from build123d import *

# Parameters (mm, degrees)
CYLINDER001_R         = 1.5
CYLINDER001_DEPTH     = 10
SKETCH002_W           = 15
SKETCH002_H           = 26
PAD_DEPTH             = 10
CLONE_SCALE_SCALE     = 2
CLONE_PLACEMENT_ANGLE = 90
BOX_W                 = 6
BOX_H                 = 20
BOX_DEPTH             = 10


with BuildPart() as obj1:
    # Cylinder001 → Cylinder001 (new body)
    with BuildSketch(Plane.XY.offset(114)):
        Circle(CYLINDER001_R)
    extrude(amount=CYLINDER001_DEPTH)


with BuildPart() as nul:
    # Sketch002 → Pad (new body)
    with BuildSketch(Plane.XY.offset(11.4)):
        with BuildLine():
            Line((-10, -18), (10, -18))
            ThreePointArc((12.5, -20.5), (11.767767, -18.732233), (10, -18))
            Line((12.5, -20.5), (12.5, -51.5))
            ThreePointArc((10, -54), (11.767767, -53.267767), (12.5, -51.5))
            Line((10, -54), (-10, -54))
            ThreePointArc((-12.5, -51.5), (-11.767767, -53.267767), (-10, -54))
            Line((-12.5, -51.5), (-12.5, -20.5))
            ThreePointArc((-10, -18), (-11.767767, -18.732233), (-12.5, -20.5))
        make_face()
        with Locations((0, -36)):
            Rectangle(SKETCH002_W, SKETCH002_H, mode=Mode.SUBTRACT)
    extrude(amount=PAD_DEPTH)


with BuildPart() as nul_1:
    # Clone scale: moved
    add(nul.part.scale(CLONE_SCALE_SCALE))


with BuildPart() as nul_2:
    # Clone placement: moved
    add(nul_1.part.moved(Location((0, 32.76, 157.8))).rotate(Axis((0, 32.76, 157.8), (1, 0, 0)), CLONE_PLACEMENT_ANGLE))


with BuildPart() as obj2:
    # Box → Box (new body)
    with BuildSketch(Plane(origin=(-3, -10, 40), x_dir=(1, 0, 0), z_dir=(0, 0, 1))):
        with Locations((3, 10)):
            Rectangle(BOX_W, BOX_H)
    extrude(amount=BOX_DEPTH)

    # Fusion001: union Nul
    add(nul_2.part)

    # Cut001: cut obj1
    add(obj1.part, mode=Mode.SUBTRACT)


solid = obj2.part
The model under review builds one solid part; all positions refer to its coordinate system, in mm. A direction names the side the tool comes from. Coordinates: 2 decimals unless noted, no trailing zeros. Loops run counter-clockwise (first coordinate to the right, second up) from the corner with the lowest first, then second, coordinate; pieces in that order, holes last.
(1) Consider section B-B, the plane y = 0. Give the boundary of the cut face in (x, z), plus the area to 3 significant figures.
Determined:
outline: (-25, 54.8) arc R5 ccw to (-20, 49.8) - (-3, 49.8) - (-3, 40) - (3, 40) - (3, 49.8) - (20, 49.8) arc R5 ccw to (25, 54.8) - (25, 116.8) arc R5 ccw to (20, 121.8) - (1.5, 121.8) - (1.5, 114) - (-1.5, 114) - (-1.5, 121.8) - (-20, 121.8) arc R5 ccw to (-25, 116.8) - close; hole (-15, 59.8) - (15, 59.8) - (15, 111.8) - (-15, 111.8) - close
area: 2,050 mm2
(2) Wall thickness on L1, parallel to Y at x = 0, z = 116.25; L2, parallel to Z at x = -14, y = 7.5; L3, parallel to Z at x = 0.5, y = 9: over which ranges is each line inside the solid? List them lowest first.
Determined:
L1: y = -10.04 to -1.5, 1.5 to 9.96
L2: z = 49.8 to 59.8, 111.8 to 121.8
L3: z = 40 to 59.8, 111.8 to 121.8
(3) Draft analysis for pull direction Z (two halves, no side actions). For faces 4 (the flat face through (0, 0, 40)), 5 (the flat face through (3, 0, 45)), 6 (the flat face through (15, 0, 85)), state which applies: +Z half, -Z half, draft (parallel to the pull), parting line (faces both ways), or undercut.
Determined:
face 4: -Z half
face 5: draft
face 6: undercut
(4) Consider section A-A, the plane x = 0. Give the boundary of the cut face in (y, z).
Determined:
outline: (-10.04, 49.8) - (-10, 49.8) - (-10, 40) - (10, 40) - (10, 50) - (9.96, 50) - (9.96, 59.8) - (-10.04, 59.8) - close; (-10.04, 111.8) - (9.96, 111.8) - (9.96, 121.8) - (1.5, 121.8) - (1.5, 114) - (-1.5, 114) - (-1.5, 121.8) - (-10.04, 121.8) - close
(5) Insertion check: P1, Ø3, axis at x = 1, z = 46.5, coming from the -Y side; P2, Ø1.8, axis at x = 0, y = 0, coming from the +Z side; P3, Ø3, axis at y = 1.5, z = 45.5, coming from the +X side. Each pin has a flat end and moves straight along its axis. Give the tip position at first contact, or say it passes through.
Determined:
P1: stops at y = -10
P2: stops at z = 114
P3: stops at x = 3
(6) Consider section D-D, the plane x = -11. Give the boundary of the cut face in (y, z).
Determined:
outline: (-10.04, 49.8) - (9.96, 49.8) - (9.96, 59.8) - (-10.04, 59.8) - close; (-10.04, 111.8) - (9.96, 111.8) - (9.96, 121.8) - (-10.04, 121.8) - close
(7) Consider section C-C, the plane z = 94. Give the boundary of the cut face in (x, y).
Determined:
outline: (-25, -10.04) - (-15, -10.04) - (-15, 9.96) - (-25, 9.96) - close; (15, -10.04) - (25, -10.04) - (25, 9.96) - (15, 9.96) - close
(8) Tool access review of faces 1 (the cylindrical face through (23.57, 0.1, 120.3)), 2 (the flat face through (0, 0, 114)), 3 (the flat face through (-15, 0, 85)): name each direction out of +Z, -Z, +X, -X, +Y, -Y from which nothing blocks a thin tool from reaching the whole face with its end or side.
Determined:
face 1: +Z, +X, +Y, -Y
face 2: +Z
face 3: +Y, -Y
